from build123d import *

# Parameters (mm, degrees)
F1_DEPTH = 25.4
F2_R     = 7.692032
F3_DEPTH = 25.4
F5_R     = 2.696649
F5_R_2   = 3.774417
F5_R_3   = 3.413238
F6_DEPTH = 25.4


with BuildPart() as f1:
    # F0 (on Top) → F1 (new body)
    with BuildSketch(Plane.XY):
        Polygon((20.889619, 24.00038), (0, 0), (44.420268, 0), (44.420268, 15.078895), (39.012816, 24.00038), align=None)
    extrude(amount=-F1_DEPTH)

    # F2 (on face) → F3 (cut)
    with BuildSketch(Plane(origin=(0, 0, -25.4), x_dir=(1, 0, 0), z_dir=(0, 0, -1))):
        with Locations((27.78032, -10.206683)):
            Circle(F2_R)
    extrude(amount=-F3_DEPTH, mode=Mode.SUBTRACT)

    # F5 (on face) → F6 (cut)
    with BuildSketch(Plane.XY):
        with Locations((35.97071, 20.118631)):
            Circle(F5_R)
        with Locations((39.374083, 9.826504)):
            Circle(F5_R_2)
        with Locations((12.639156, 5.767059)):
            Circle(F5_R_3)
    extrude(amount=-F6_DEPTH, mode=Mode.SUBTRACT)


solid = f1.part
Input: part model. Units: mm. Frame: model coordinates. Give positions to 0.01 mm unless a question says otherwise; leave off trailing zeros. Order: outer loops, then holes, each group sorted by start corner. A loop starts at its lowest first (then second) coordinate and runs counter-clockwise, first axis right, second up. Notation, with made-up numbers: M 3,58 L 27,58 A21 cw 27,74 Z; hole C 46,34.5 d7. An arc over 180 degrees is marked long. Answer as a JSON object with one key per item and string values.
1. First-contact query: P1, Ø10, axis at x = 17.5, z = -9.5, coming from the +Y side; P2, Ø7, axis at x = 39.37, y = 9.83, coming from the -Z side. Flat tips, straight axial feed; report the tip coordinate or a pass-through.
Result sheet:
{"P1": "y = 24", "P2": "through"}
2. Cut plane D-D, the plane z = -21. Output: boundary loops of the cut face in (x, y), and give its area (3 significant figures).
Result sheet:
{"outline": "M 0,0 L 44.42,0 L 44.42,15.08 L 39.01,24 L 20.89,24 Z; hole C 12.64,5.77 d6.83; hole C 27.78,10.21 d15.38; hole C 35.97,20.12 d5.39; hole C 39.37,9.83 d7.55", "area": "501 mm²"}
3. Pull-direction query (X, two-part tool) for faces 1 (the cylindrical face through (22.11, 5.01, -12.88)), 2 (the flat face through (10.59, 12.17, -12.52)), 3 (the flat face through (41.754, 19.477, -12.522)); classes: +X half, -X half, draft (parallel to the pull), parting line (faces both ways), or undercut.
Result sheet:
{"face 1": "undercut", "face 2": "-X half", "face 3": "+X half"}
4. Cut plane A-A, the plane x = 30. Output: boundary loops of the cut face in (y, z), and give its area (3 significant figures).
Result sheet:
{"outline": "M 0,-25.4 L 2.84,-25.4 L 2.84,0 L 0,0 Z; M 17.57,-25.4 L 24,-25.4 L 24,0 L 17.57,0 Z", "area": "235 mm²"}
5. Ray query, line 1 (X direction, y = 5.5, z = -7.5); line 2 (X direction, y = 4.5, z = -23.25); line 3 (Y direction, x = 34, z = -15.25). Return the intervals inside material, ascending. Write a range as [from, to].
Result sheet:
{"line 1": "[4.79, 9.24], [16.04, 21.7], [33.86, 44.42]", "line 2": "[3.92, 9.47], [15.81, 22.62], [32.94, 44.42]", "line 3": "[0, 5.68], [14.73, 18.28], [21.96, 24]"}
6. Cut plane C-C, the plane y = 4.75. Output: boundary loops of the cut face in (x, z).
Result sheet:
{"outline": "M 4.13,-25.4 L 9.38,-25.4 L 9.38,0 L 4.13,0 Z; M 15.9,-25.4 L 22.36,-25.4 L 22.36,0 L 15.9,0 Z; M 33.2,-25.4 L 44.42,-25.4 L 44.42,0 L 33.2,0 Z"}
7. Cut plane B-B, the plane y = 7.5. Output: boundary loops of the cut face in (x, z), and give its area (3 significant figures).
Result sheet:
{"outline": "M 6.53,-25.4 L 9.7,-25.4 L 9.7,0 L 6.53,0 Z; M 15.58,-25.4 L 20.58,-25.4 L 20.58,0 L 15.58,0 Z; M 34.98,-25.4 L 36.4,-25.4 L 36.4,0 L 34.98,0 Z; M 42.35,-25.4 L 44.42,-25.4 L 44.42,0 L 42.35,0 Z", "area": "296 mm²"}
